Geometry: final body of the model. Coordinates: model frame, mm. Coordinates: 2 decimals unless noted, no trailing zeros. Loops run counter-clockwise (first coordinate to the right, second up) from the corner with the lowest first, then second, coordinate; pieces in that order, holes last. Notation, with made-up numbers: M -4,-24 L 48,-24 A10 ccw 48,-10 Z; hole C 56,-20.75 d10. An arc over 180 degrees is marked long. Write each question's results on one line, items separated by ' | '. Start each with the question number.
Autodesk Inventor part; units mm, degrees
ref_plane "YZ Plane" through (0, 0, 0) normal (1, 0, 0) x (0, 1, 0)
ref_plane "XZ Plane" through (0, 0, 0) normal (0, 1, 0) x (-1, 0, 0)
ref_plane "XY Plane" through (0, 0, 0) normal (0, 0, 1) x (1, 0, 0)
sketch "Sketch1" plane through (0, 0, 0) normal (0, 1, 0) x (-1, 0, 0)
  circle A0 centre (0, 0) radius 1.5
  dimension "d0" = 3
extrude "Extrusion1" add sketch "Sketch1" along normal blind 20
sketch "Sketch2" plane through (0, 20, 0) normal (0, 1, 0) x (1, 0, 0)
  circle A0 centre (0, 0) radius 2.5
  dimension "d3" = 5
extrude "Extrusion2" add sketch "Sketch2" along normal blind 2
fillet "Fillet1" radius 1.7 1 edges at (-2.5, 22, 0)
chamfer "Chamfer1" distance 0.3 angle 45 1 edges at (1.5, 0, 0)
thread "Thread1"
sketch "Sketch3" plane through (0, 22, 0) normal (0, 1, 0) x (1, 0, 0)
  line L0 (0.5, -2.5) -> (0.5, 2.5)
  line L1 (0.5, 2.5) -> (-0.5, 2.5)
  line L2 (-0.5, 2.5) -> (-0.5, -2.5)
  line L3 (-0.5, -2.5) -> (0.5, -2.5)
  line L4 (0.5, -2.5) -> (-0.5, 2.5) construction
  line L5 (0.5, 2.5) -> (-0.5, -2.5) construction
  line L6 (1.5, -0.5) -> (-1.5, -0.5)
  line L7 (-1.5, -0.5) -> (-1.5, 0.5)
  line L8 (-1.5, 0.5) -> (1.5, 0.5)
  line L9 (1.5, 0.5) -> (1.5, -0.5)
  circle A0 centre (0, 0) radius 2.5
  line L10 (1.5, -0.5) -> (-1.5, 0.5) construction
  line L11 (-1.5, -0.5) -> (1.5, 0.5) construction
  dimension "d12" = 1
  dimension "d13" = 3
  dimension "d14" = 1
extrude "Extrusion3" cut sketch "Sketch3" against normal blind 0.7 contours L3 A0 L0 | A0 L2 L6 L0 | L3 L2 A0 | L6 L2 L8 L0 | L0 L8 L9 L6 | L8 L2 A0 L0 | L6 L7 L8 L2 | A0 L1 L0 | L2 L1 A0
properties part number "M3x10 Screw Nylon" material "Steel"
Item 1: Contact query for flat-ended pins moving along their axis: P1, Ø0.6, axis at x = 1, y = 21.5, coming from the +Z side; P2, Ø0.8, axis at y = 21.5, z = 1, coming from the +X side; P3, Ø1, axis at x = -1, y = 18.5, coming from the -Z side. Output: stop coordinate, or through.
Item 2: Pull-direction query (X, two-part tool) for faces 1 (the flat face through (0, 21.3, 0)), 2 (the flat face through (0, 0, 0)), 3 (the cylindrical face through (1.15, 20.15, -2.22)); classes: released by +X, released by -X, zero draft, split by the parting line, or undercut.
Item 3: Section A-A, the plane y = 7.5. Return loops of the section in (x, z), plus the area to 3 significant figures.
Item 4: Ray query, L1, parallel to Y at x = 0.5, z = 0.4; L2, parallel to Y at x = -0.05, z = 2.15; L3, parallel to Z at x = 0.05, y = 19.75. Return the intervals inside material, ascending. Write a range as [from, to].
Solutions:
1) P1: stops at z = 2.05 | P2: stops at x = 2.12 | P3: stops at z = -1.41
2) face 1: undercut | face 2: zero draft | face 3: split by the parting line
3) outline: C 0,0 d3 | area: 7.07 mm²
4) L1: y = [0, 21.3] | L2: y = [20, 21.3] | L3: z = [-1.5, 1.5]
